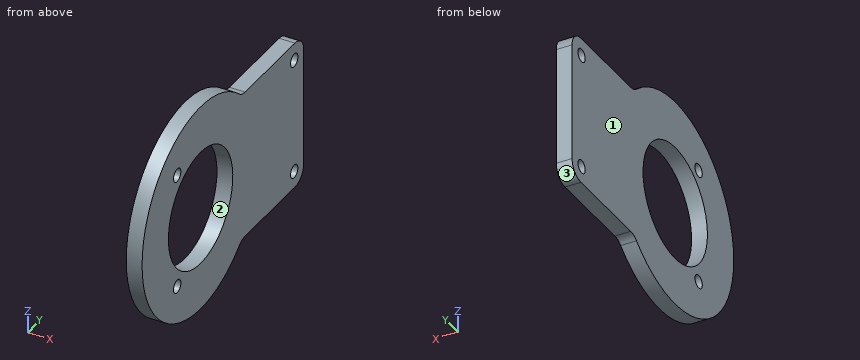
Autodesk Inventor part; units mm, degrees
ref_plane "YZ Plane" through (0, 0, 0) normal (1, 0, 0) x (0, 1, 0)
ref_plane "XZ Plane" through (0, 0, 0) normal (0, 1, 0) x (-1, 0, 0)
ref_plane "XY Plane" through (0, 0, 0) normal (0, 0, 1) x (1, 0, 0)
sketch "スケッチ1" plane through (0, 0, 0) normal (1, 0, 0) x (0, 1, 0)
  circle A0 centre (0, 0) radius 20
  line L0 (0, 0) -> (35.25, 0)
  line L1 (35.25, 0) -> (35.25, -14.25)
  line L2 (35.25, -14.25) -> (0, -14.25)
  line L3 (0, -14.25) -> (0, 0)
  line L4 (35.25, 0) -> (35.25, 14.25)
  line L5 (35.25, 14.25) -> (0, 14.25)
  point P0 (14.0334, 14.25)
  point P1 (14.0334, -14.25)
  dimension "d0" = 40
  dimension "d1" = 14.25
  dimension "d2" = 35.25
extrude "押し出し1" add sketch "スケッチ1" along normal blind 3
sketch "スケッチ2" plane through (3, 0, 0) normal (1, 0, 0) x (0, 0, -1)
  line L0 (14.25, 35.25) -> (-14.25, 35.25)
  line L1 (-14.25, 35.25) -> (14.25, 35.25)
  line L2 (14.25, 35.25) -> (14.25, -11.25)
  line L3 (14.25, -11.25) -> (-14.25, -11.25)
  line L4 (-14.25, -11.25) -> (-14.25, 35.25)
  line L5 (-11, 32) -> (11, 32)
  line L6 (11, 32) -> (11, -8)
  line L7 (11, -8) -> (-11, -8)
  line L8 (-11, -8) -> (-11, 32)
  point P0 (0, 0)
  dimension "d5" = 46.5
  dimension "d6" = 3.25
  dimension "d7" = 3.25
  dimension "d8" = 3.25
  dimension "d9" = 3.25
hole "穴1" at (3, -8, 11) at (3, -8, -11) at (3, 32, -11) at (3, 32, 11) direction (-1, 0, 0) diameter 2.5 end through all
sketch "スケッチ3" plane through (0, 0, 0) normal (-1, 0, 0) x (0, 0, 1)
  circle A0 centre (0, 0) radius 11
  dimension "d17" = 22
extrude "押し出し2" cut sketch "スケッチ3" against normal blind 3
fillet "フィレット1" radius 3 4 edges at (1.5, 35.25, 14.25) (1.5, 14.0334, 14.25) (1.5, 35.25, -14.25) (1.5, 14.0334, -14.25)
properties part number "connectplate4" material "アルミニウム 6061"
Geometry: final body of the model. Coordinates: model frame, mm. Face numbers are marked on the shaded views. Give positions to 0.01 mm unless a question says otherwise; leave off trailing zeros. Order: outer loops, then holes, each group sorted by start corner. A loop starts at its lowest first (then second) coordinate and runs counter-clockwise, first axis right, second up. Notation, with made-up numbers: (76, 86) -> (92, 86) arc R34 ccw to (92, 118) -> close; hole circle Ø11 at (5.25, 82). An arc over 180 degrees is marked (long way). Write each question's results on one line, items separated by ' | '.
1) Draft query along Y for the marked faces 1, 2 and 3. Return one class per face: released by +Y, released by -Y, zero draft, split by the parting line, or undercut.
Geometry says:
face 1: zero draft | face 2: undercut | face 3: released by +Y
2) Line query: line 1 along Z through (x, y) = (1.6, 32); line 2 along Y through (x, z) = (2.45, 12); line 3 along Y through (x, z) = (2.3, 0). Output: solid intervals per line, ascending.
Geometry says:
line 1: z = -14.25 to -12.25, -9.75 to 9.75, 12.25 to 14.25 | line 2: y = -16 to -8.75, -7.25 to 31.25, 32.75 to 35.15 | line 3: y = -20 to -11, 11 to 35.25
3) First-contact query: pin 1 Ø6 at (y, z) = (-6.5, 15.5) entering from -X; pin 2 Ø1.5 at (x, y) = (1.5, 20.5) entering from -Z; pin 3 Ø1 at (x, y) = (2, 22.5) entering from +Z. Flat tips, straight axial feed; report the tip coordinate or a pass-through.
Geometry says:
pin 1: stops at x = 0 | pin 2: stops at z = -14.25 | pin 3: stops at z = 14.25
4) Cut plane B-B (x = 1.95). Output: boundary loops of the cut face in (y, z).
Geometry says:
outline: (13.23, -15) arc R3 cw to (15.21, -14.25) -> (32.25, -14.25) arc R3 ccw to (35.25, -11.25) -> (35.25, 11.25) arc R3 ccw to (32.25, 14.25) -> (15.21, 14.25) arc R3 cw to (13.23, 15) arc R20 ccw (long way) to start; hole circle Ø22 at (0, 0); hole circle Ø2.5 at (-8, -11); hole circle Ø2.5 at (-8, 11); hole circle Ø2.5 at (32, -11); hole circle Ø2.5 at (32, 11)
5) Cut plane C-C (y = -8). Output: boundary loops of the cut face in (x, z), and give its area (3 significant figures).
Geometry says:
outline: (0, -18.33) -> (3, -18.33) -> (3, -12.25) -> (0, -12.25) -> close; (0, -9.75) -> (3, -9.75) -> (3, -7.55) -> (0, -7.55) -> close; (0, 7.55) -> (3, 7.55) -> (3, 9.75) -> (0, 9.75) -> close; (0, 12.25) -> (3, 12.25) -> (3, 18.33) -> (0, 18.33) -> close | area: 49.7 mm²
6) Cut plane D-D (y = 4.5). Output: boundary loops of the cut face in (x, z), and give its area (3 significant figures).
Geometry says:
outline: (0, -19.49) -> (3, -19.49) -> (3, -10.04) -> (0, -10.04) -> close; (0, 10.04) -> (3, 10.04) -> (3, 19.49) -> (0, 19.49) -> close | area: 56.7 mm²
7) Cut plane A-A (z = 0). Output: boundary loops of the cut face in (x, y), and give its area (4 significant figures).
Geometry says:
outline: (0, -20) -> (3, -20) -> (3, -11) -> (0, -11) -> close; (0, 11) -> (3, 11) -> (3, 35.25) -> (0, 35.25) -> close | area: 99.75 mm²
